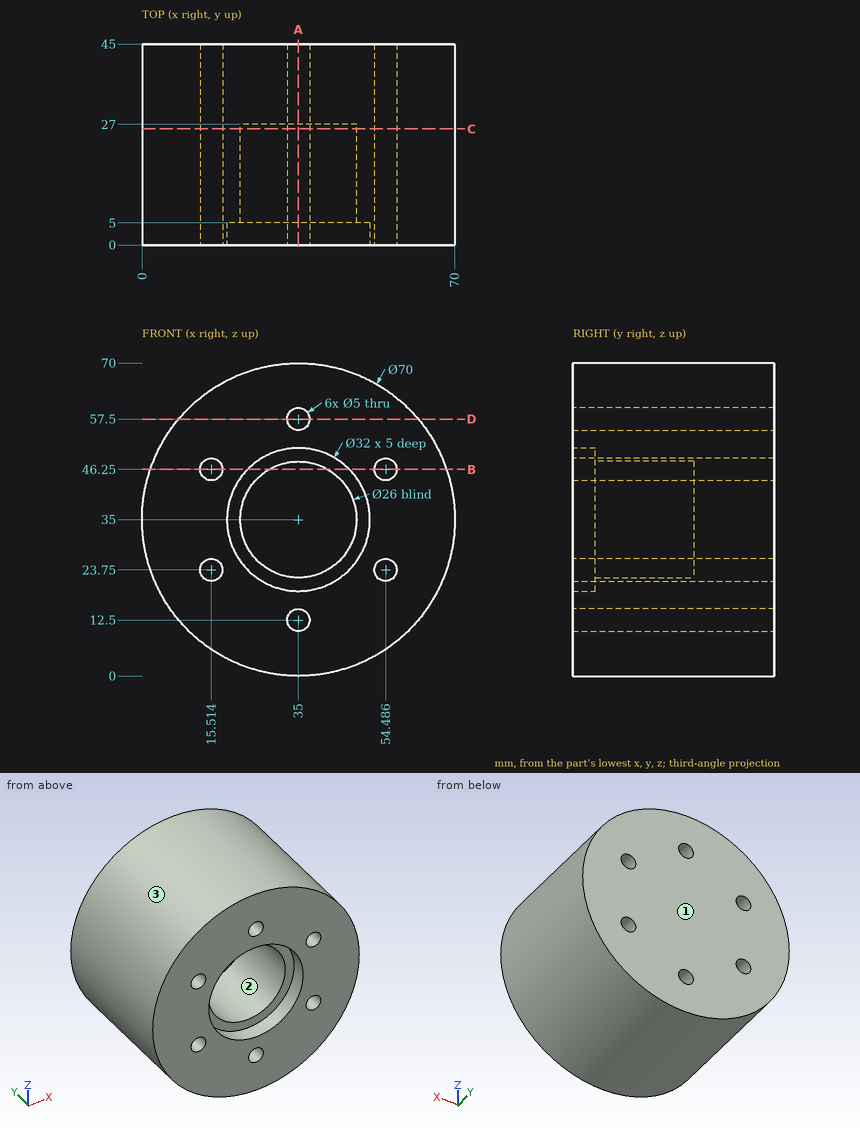
Can you work these out from the drawing? Everything is in mm from the part's minimum corner. Coordinates: 2 decimals unless noted, no trailing zeros. Write each loop counter-clockwise with the first axis right and the second up, starting at its lowest first coordinate (ties: lowest second). Pieces come first, ordered by that corner, then holes. Notation, with made-up numbers: (-13.75, 89.25) -> (-4.75, 89.25) arc R13 ccw to (-4.75, 93.25) -> close; hole circle Ø1 at (-7.5, -7). An arc over 180 degrees is marked (long way). Return JSON: item names as keys, results as strings.
(1) Imagine slicing it at D-D, the plane z = 57.5. Please give me the cut outline in (x, y), then the cut area to 3 significant figures.
Numbers:
{"outline": "(8.19, 0) -> (32.5, 0) -> (32.5, 45) -> (8.19, 45) -> close; (37.5, 0) -> (61.81, 0) -> (61.81, 45) -> (37.5, 45) -> close", "area": "2,190 mm2"}
(2) Imagine slicing it at C-C, the plane y = 26. Count the separate pieces of the cut face and the enclosed holes in it, then the cut area to 3 significant figures.
Numbers:
{"separate pieces": "1", "enclosed holes": "7", "area": "3,200 mm2"}
(3) I'm going to push flat-ended pins straight in: pin 1 (2 mm diameter, centred on y = 36, z = 42, fed in from -X); pin 2 (4 mm diameter, centred on y = 17.5, z = 13, fed in from +X); pin 3 (10 mm diameter, centred on x = 49, y = 33.5, fed in from -Z); pin 4 (3 mm diameter, centred on x = 15.51, z = 23.75, fed in from +Y). Where does each tip first touch, or does it pass through?
Numbers:
{"pin 1": "stops at x = 0.52", "pin 2": "stops at x = 63.72", "pin 3": "stops at z = 1.18", "pin 4": "passes through"}
(4) We'd pull the mould along Z, two halves only. Please class the marked faces 1, 2 and 3: +Z half, -Z half, draft (parallel to the pull), parting line (faces both ways), or undercut.
Numbers:
{"face 1": "draft", "face 2": "undercut", "face 3": "parting line"}
(5) Imagine slicing it at B-B, the plane z = 46.25. Please give me the cut outline in (x, y) (1 decimal), then the cut area to 3 significant figures.
Numbers:
{"outline": "(1.9, 0) -> (13, 0) -> (13, 45) -> (1.9, 45) -> close; (18, 0) -> (23.6, 0) -> (23.6, 5) -> (28.5, 5) -> (28.5, 27) -> (41.5, 27) -> (41.5, 5) -> (46.4, 5) -> (46.4, 0) -> (52, 0) -> (52, 45) -> (18, 45) -> close; (57, 0) -> (68.1, 0) -> (68.1, 45) -> (57, 45) -> close", "area": "2,130 mm2"}
(6) I need wall thicknesses on L1, parallel to Z at x = 55, y = 5.5 (1 decimal); L2, parallel to X at y = 3.6, z = 35; L3, parallel to Z at x = 53, y = 29.5 (1 decimal). Which ranges of each line are inside material? Lowest first, please.
Numbers:
{"L1": "z = 6.3 to 21.3, 26.2 to 43.8, 48.7 to 63.7", "L2": "x = 0 to 19, 51 to 70", "L3": "z = 5 to 21.7, 25.8 to 44.2, 48.3 to 65"}
(7) Imagine slicing it at A-A, the plane x = 35. Please give me the cut outline in (y, z).
Numbers:
{"outline": "(0, 0) -> (45, 0) -> (45, 10) -> (0, 10) -> close; (0, 15) -> (45, 15) -> (45, 55) -> (0, 55) -> (0, 51) -> (5, 51) -> (5, 48) -> (27, 48) -> (27, 22) -> (5, 22) -> (5, 19) -> (0, 19) -> close; (0, 60) -> (45, 60) -> (45, 70) -> (0, 70) -> close"}
